Verification items for the finished model (mm, model axes). Face numbers are marked on the shaded views. A direction names the side the tool comes from. Coordinates: 2 decimals unless noted, no trailing zeros. Write each loop counter-clockwise with the first axis right and the second up, starting at its lowest first coordinate (ties: lowest second). Pieces come first, ordered by that corner, then holes. Notation, with made-up numbers: M 85,58.25 L 111,58.25 A7 cw 111,63.25 Z; hole C 8.5,86.25 d5. An arc over 180 degrees is marked long. Answer in a Markdown table with one row per item.
from build123d import *

# Parameters (mm, degrees)
F0_W     = 42
F0_H     = 40
F0_R     = 6.25
F1_DEPTH = 10
F2_SIZE  = 10
F4_D     = 4.5
F6_D     = 6.6
F6_DEPTH = 10
F6_TIP   = 1.9828400428


with BuildPart() as f1:
    # F0 (on Front) → F1 (new body)
    with BuildSketch(Plane.XZ):
        Rectangle(F0_W, F0_H)
        with Locations((6, 0)):
            Circle(F0_R, mode=Mode.SUBTRACT)
    extrude(amount=F1_DEPTH)

    # F2
    f2_edges = [f1.edges().sort_by_distance(p)[0] for p in [
        (21, -5, 20),
        (21, -5, -20),
    ]]
    chamfer(f2_edges, length=F2_SIZE)

    # F4 (through all)
    with Locations(Plane.XZ.offset(10)):
        with Locations((-1, 7), (-1, -7), (13, -7), (13, 7)):
            Hole(F4_D / 2)

    # F6
    with Locations(Plane(origin=(-21, 0, 0), x_dir=(0, -1, 0), z_dir=(-1, 0, 0))):
        with Locations((5, 15), (5, -15)):
            Hole(F6_D / 2, depth=F6_DEPTH)
            with Locations((0, 0, -(F6_DEPTH + F6_TIP / 2))):  # 118° drill point
                Cone(0, F6_D / 2, F6_TIP, mode=Mode.SUBTRACT)


solid = f1.part
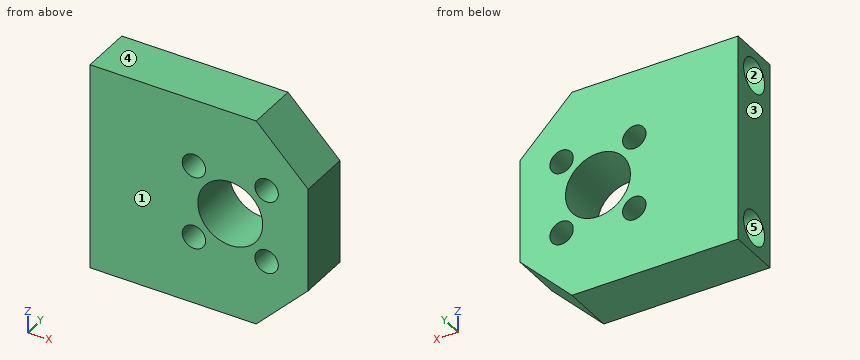
1) Sectioned sample at D-D (x = 6). Record the cut outline in (y, z), then the cut area to 3 significant figures.
Response values:
| item | result |
|---|---|
| outline | M -10,-20 L 0,-20 L 0,-6.25 L -10,-6.25 Z; M -10,6.25 L 0,6.25 L 0,20 L -10,20 Z |
| area | 275 mm² |
2) Sectioned sample at B-B (x = -1). Record the cut outline in (y, z), then the cut area to 3 significant figures.
Response values:
| item | result |
|---|---|
| outline | M -10,-20 L 0,-20 L 0,-9.25 L -10,-9.25 Z; M -10,-4.75 L 0,-4.75 L 0,4.75 L -10,4.75 Z; M -10,9.25 L 0,9.25 L 0,20 L -10,20 Z |
| area | 310 mm² |
3) Thickness scan on L1, parallel to Z at x = -1, y = -7; L2, parallel to Z at x = -14, y = -5; L3, parallel to Y at x = -15.75, z = 15. Record the ranges inside material, lowest first. Write a range as [from, to].
Response values:
| item | result |
|---|---|
| L1 | z = [-20, -9.25], [-4.75, 4.75], [9.25, 20] |
| L2 | z = [-20, -18.3], [-11.7, 11.7], [18.3, 20] |
| L3 | y = [-10, -8.3], [-1.7, 0] |
4) Sectioned sample at C-C (z = 0). Record the cut outline in (x, y), then the cut area to 3 significant figures.
Response values:
| item | result |
|---|---|
| outline | M -21,-10 L -0.25,-10 L -0.25,0 L -21,0 Z; M 12.25,-10 L 21,-10 L 21,0 L 12.25,0 Z |
| area | 295 mm² |
5) Release check for a two-part mould opening along Y. For the marked faces 1, 2 and 3 record: +Y half, -Y half, draft (parallel to the pull), parting line (faces both ways), or undercut.
Response values:
| item | result |
|---|---|
| face 1 | -Y half |
| face 2 | undercut |
| face 3 | draft |
6) Tool access check on the marked faces 4 and 5. Record the directions out of +Z, -Z, +X, -X, +Y, -Y that give a thin tool (end or side, any length) a straight path to the whole face; none if there is none.
Response values:
| item | result |
|---|---|
| face 4 | +Z, +X, -X, +Y, -Y |
| face 5 | -X |
7) Depth check by flat-ended pin: pin 1 (5 mm diameter, centred on x = -1, z = -7, fed in from +Y); pin 2 (4 mm diameter, centred on y = -2.5, z = 16, fed in from +X); pin 3 (5.5 mm diameter, centred on y = -5, z = 15, fed in from -X); pin 4 (4 mm diameter, centred on x = 13, z = 7, fed in from +Y). Enter the tip coordinate at first touch or a pass-through.
Response values:
| item | result |
|---|---|
| pin 1 | stops at y = 0 |
| pin 2 | stops at x = 17 |
| pin 3 | stops at x = -10.67 |
| pin 4 | passes through |
8) Sectioned sample at A-A (z = 7). Record the cut outline in (x, y).
Response values:
| item | result |
|---|---|
| outline | M -21,-10 L -3.25,-10 L -3.25,0 L -21,0 Z; M 1.25,-10 L 10.75,-10 L 10.75,0 L 1.25,0 Z; M 15.25,-10 L 21,-10 L 21,0 L 15.25,0 Z |
